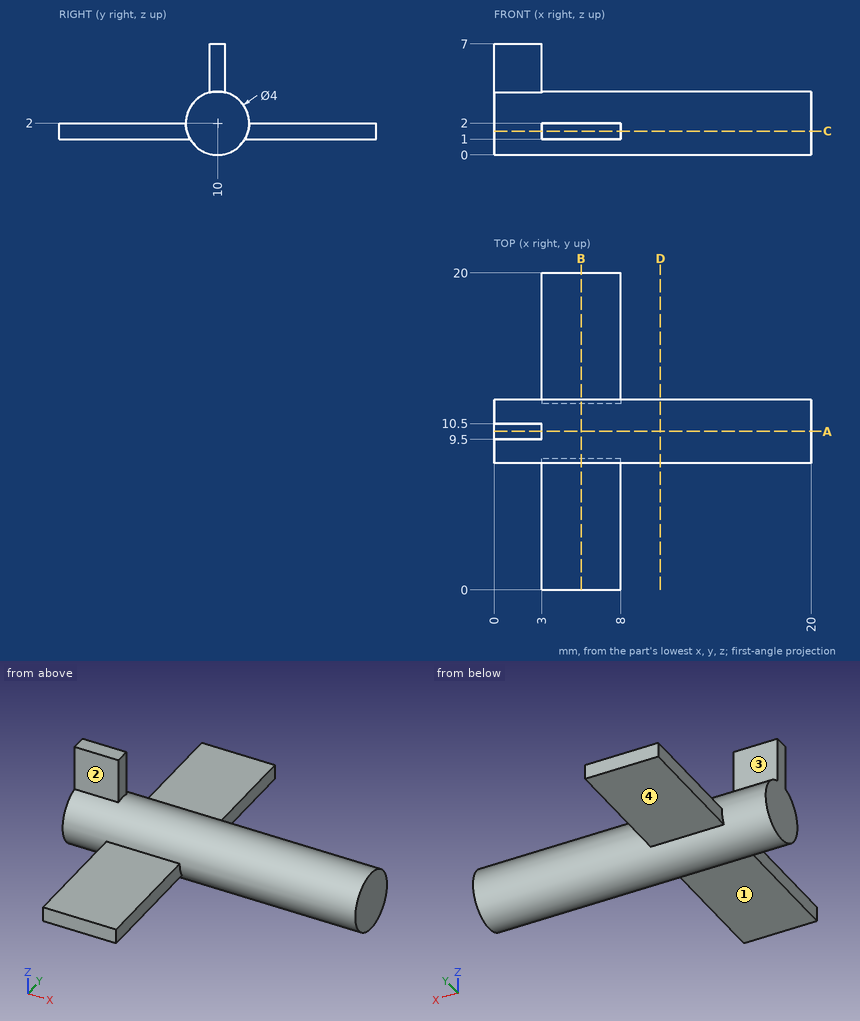
Print and shaded views of the part. All mm, measured from the part's lowest x, y and z. A direction names the side the tool comes from. Round coordinates to 2 decimals unless told otherwise and drop trailing zeros. Write each loop counter-clockwise with the first axis right and the second up, starting at its lowest first coordinate (ties: lowest second). Pieces come first, ordered by that corner, then holes.
(1) Slice it at C-C, the plane z = 1.5. Write the cut outline in (x, y).
(2) 3-axis set-ups, long thin cutter, end or side, ignore diameter. For the marked faces 1, 2, 3 and 4: which of +Z, -Z, +X, -X, +Y, -Y reach the whole face in a straight line?
(3) Slice it at A-A, the plane y = 10. Write the cut outline in (x, z), and give its area (3 significant figures).
(4) Probe line 1 along Z through (x, y) = (5.5, 14); line 2 along X through (y, z) = (19.25, 1.75); line 3 along Y through (x, z) = (18.5, 2.5). List the from-to ranges inside material, lowest first.
(5) Drop flat-ended pins along their axis: P1, Ø0.5, axis at y = 16, z = 1.5, coming from the +X side; P2, Ø0.9, axis at x = 1.5, z = 5.5, coming from the -Y side; P3, Ø0.8, axis at y = 5.5, z = 1.5, coming from the -X side; P4, Ø2, axis at y = 10.5, z = 2.5, coming from the -X side. Give the stop position or say it passes through.
(6) Slice it at D-D, the plane x = 10.5. Write the cut outline in (y, z).
(7) Slice it at B-B, the plane x = 5.5. Write the cut outline in (y, z), and give its area (3 significant figures).
From the geometry:
1. outline: (0, 8.06) - (3, 8.06) - (3, 0) - (8, 0) - (8, 8.06) - (20, 8.06) - (20, 11.94) - (8, 11.94) - (8, 20) - (3, 20) - (3, 11.94) - (0, 11.94) - close
2. face 1: -Z, +X, -X, -Y
2. face 2: +Z, +X, -X, -Y
2. face 3: +Z, +X, -X, +Y
2. face 4: -Z, +X, -X, +Y
3. outline: (0, 0) - (20, 0) - (20, 4) - (3, 4) - (3, 7) - (0, 7) - close
3. area: 89.0 mm2
4. line 1: z = 1 to 2
4. line 2: x = 3 to 8
4. line 3: y = 8.06 to 11.94
5. P1: stops at x = 8
5. P2: stops at y = 9.5
5. P3: stops at x = 3
5. P4: stops at x = 0
6. outline: circle Ø4 at (10, 2)
7. outline: (0, 1) - (8.27, 1) arc R2 ccw to (11.73, 1) - (20, 1) - (20, 2) - (12, 2) arc R2 ccw to (8, 2) - (0, 2) - close
7. area: 28.7 mm2
